Autodesk Inventor part; units mm, degrees
ref_plane "YZ Plane" through (0, 0, 0) normal (1, 0, 0) x (0, 1, 0)
ref_plane "XZ Plane" through (0, 0, 0) normal (0, 1, 0) x (-1, 0, 0)
ref_plane "XY Plane" through (0, 0, 0) normal (0, 0, 1) x (1, 0, 0)
sketch "Sketch1" plane through (0, 0, 0) normal (0, 0, 1) x (1, 0, 0)
  arc A0 (-375.92, 0) -> (187.96, -325.5563) centre (0, 0) ccw
  arc A1 (-378.46, 0) -> (189.23, -327.756) centre (0, 0) ccw
  line L0 (0, 0) -> (189.23, -327.756)
  line L1 (0, 0) -> (-378.46, 0)
  line L2 (-378.46, 0) -> (-378.46, -78.74)
  line L3 (-378.46, -78.74) -> (-370.1783, -78.74)
  line L4 (189.23, -327.756) -> (121.0392, -367.126)
  line L5 (121.0392, -367.126) -> (116.8983, -359.9538)
  dimension "d0" = 751.84
  dimension "d1" = 756.92
  dimension "d2" = 120
  dimension "d3" = 78.74
  dimension "d4" = 78.74
extrude "Extrusion1" add sketch "Sketch1" along normal blind 76.2 contours A0 L0 A1 L1 | A1 L3 L2 | L4 L5 A1
sketch "Sketch2" plane through (121.0392, -367.126, 0) normal (0.5, -0.866, 0) x (0.866, 0.5, 0)
  line L0 (0, 0) -> (78.74, 0)
  line L1 (78.74, 0) -> (78.74, 76.2)
  point P0 (39.37, 19.05)
  point P1 (39.37, 38.1)
  point P2 (39.37, 57.15)
  dimension "d7" = 19.05
  dimension "d8" = 38.1
  dimension "d9" = 57.15
  dimension "d10" = 39.37
  dimension "d11" = 39.37
  dimension "d12" = 39.37
sketch "Sketch3" plane through (-378.46, -78.74, 0) normal (-1, 0, 0) x (0, 0, 1)
  line L0 (0, 78.74) -> (76.2, 78.74)
  line L1 (0, 78.74) -> (0, 0)
  point P0 (19.05, 39.37)
  point P1 (38.1, 39.37)
  point P2 (57.15, 39.37)
  dimension "d13" = 19.05
  dimension "d14" = 38.1
  dimension "d15" = 57.15
  dimension "d16" = 39.37
  dimension "d17" = 39.37
  dimension "d18" = 39.37
hole "Hole1" at (-378.46, -39.37, 57.15) at (-378.46, -39.37, 38.1) at (-378.46, -39.37, 19.05) direction (1, 0, 0) diameter 6.35 depth 25.4 tip angle 118
hole "Hole2" at (155.1346, -347.441, 19.05) at (155.1346, -347.441, 38.1) at (155.1346, -347.441, 57.15) direction (-0.5, 0.866, 0) diameter 6.35 depth 25.4 tip angle 118
properties part number "120 degree curved track"
CAD build for the part. Positions are in the model's coordinates, mm. Coordinates: 2 decimals unless noted, no trailing zeros. Write each loop counter-clockwise with the first axis right and the second up, starting at its lowest first coordinate (ties: lowest second). Pieces come first, ordered by that corner, then holes. Notation, with made-up numbers: (24.25, 38) -> (40.25, 38) arc R11 cw to (40.25, 51) -> close; hole circle Ø9 at (0.5, 59.5). An arc over 180 degrees is marked (long way). Return JSON: item names as keys, results as strings. Group by question number.
Q1. Cut at A-A, the plane x = -204. Give the cut face in (y, z), then the cut area to 3 significant figures.
Q2. Drill centre lines: line 1 (Z direction, x = -376, y = -39); line 2 (Y direction, x = -376, z = 38); line 3 (X direction, y = -347, z = 40.5). Where is each one in solid material? Low to high.
Q3. Flat gauge pins, fed straight in: pin 1 (4 mm diameter, centred on x = 54, z = 28, fed in from -Y); pin 2 (12 mm diameter, centred on y = -163, z = 39, fed in from +X); pin 3 (8 mm diameter, centred on y = -169.5, z = 62, fed in from -X). Where does each tip first touch, or does it go through?
Q4. Cut at B-B, the plane y = -119. Give the cut face in (x, z), then the cut area to 3 significant figures.
Returned:
{
 "1": {"outline": "(-318.77, 0) -> (-315.75, 0) -> (-315.75, 76.2) -> (-318.77, 76.2) -> close", "area": "230 mm2"},
 "2": {"line 1": "z = 0 to 15.9, 22.2 to 34.95, 41.25 to 54, 60.3 to 76.2", "line 2": "y = -78.74 to -42.54, -36.2 to 0", "line 3": "x = -151.07 to -144.59, 144.59 to 152.48"},
 "3": {"pin 1": "stops at y = -374.87", "pin 2": "stops at x = -335.79", "pin 3": "stops at x = -340.36"},
 "4": {"outline": "(-359.26, 0) -> (-356.59, 0) -> (-356.59, 76.2) -> (-359.26, 76.2) -> close", "area": "204 mm2"}
}
